Design review of the part built by this model. Coordinates are the model's own, in mm. A direction names the side the tool comes from. Coordinates: 2 decimals unless noted, no trailing zeros. Write each loop counter-clockwise with the first axis right and the second up, starting at its lowest first coordinate (ties: lowest second). Pieces come first, ordered by that corner, then holes. Notation, with made-up numbers: (11, 36) -> (51, 36) arc R10 ccw to (51, 51) -> close; hole circle Ø9 at (30.5, 79.25). An arc over 180 degrees is marked (long way). Answer in a Markdown table with one row per item. Add a question column.
Item 1: Clearance check with flat-ended pins moving along their axes: P1, Ø3.5, axis at x = 11.5, z = 6.5, coming from the -Y side; P2, Ø0.9, axis at x = -3.5, y = -0.5, coming from the -Z side; P3, Ø2, axis at x = -18.5, z = 1.5, coming from the -Y side; P4, Ø4, axis at x = -2.5, z = 1.5, coming from the -Y side. State where each tip first meets the part, or that it passes through.
Item 2: Take a section at A-A, the plane x = -11.5. Write out the cut boundary in (y, z), and give its area (3 significant figures).
Item 3: Take a section at B-B, the plane y = -1. Write out the cut boundary in (x, z).
Item 4: For faces 5 (the face through (-26, 2, 6)), 6 (the face through (-20.62, 0.44, 3.8)), 7 (the face through (-8.324, -2.958, 4.701)), list the 3-axis set-ups (+Z, -Z, +X, -X, +Y, -Y) from which the entire face can be reached by the end or side of a thin tool; tool diameter is ignored.
Item 5: Take a section at C-C, the plane z = 12.25. Write out the cut boundary in (x, y).
Item 6: Draft analysis for pull direction Z (two halves, no side actions). For faces 1 (the face through (-5, 0, 13)), 2 (the face through (-5.88, -4.9, 6.41)), 3 (the face through (11, -1, 10.15)), 4 (the face through (14.646, -1.479, 8.351)), state which applies: released by +Z, released by -Z, zero draft, split by the parting line, or undercut.
Item 7: To check wall thickness, follow line 1 (Z direction, x = -11.5, y = 1.05); line 2 (Z direction, x = 13, y = -1.5); line 3 (X direction, y = -1, z = 6.75). State the ranges of each line that lie inside material, in increasing order.
Item 8: Take a section at D-D, the plane x = 11.5. Write out the cut boundary in (y, z).
from build123d import *

# Parameters (mm, degrees)
F0_R     = 1.45
F1_DEPTH = 13
F2_R     = 2.15
F3_DEPTH = 9.001
F4_DEPTH = 3
F5_DEPTH = 7.7


with BuildPart() as f1:
    # F0 (on Top) → F1 (new body)
    with BuildSketch(Plane.XY):
        with BuildLine():
            Line((17, -3), (17, 3))
            Line((17, 3), (-26, 3))
            Line((-26, 3), (-26, 0))
            ThreePointArc((-26, 0), (-25.2642971497, -2.3117880782), (-23.3278179407, -3.7731816172))
            Line((-23.3278179407, -3.7731816172), (-17, -6))
            Line((-17, -6), (-9, -6))
            Line((-9, -6), (-2.6721820593, -3.7731816172))
            ThreePointArc((-2.6721820593, -3.7731816172), (-1.9759531619, -3.4501064327), (-1.3542486889, -3))
            Line((-1.3542486889, -3), (17, -3))
        make_face()
        with Locations((-22, 0)):
            Circle(F0_R, mode=Mode.SUBTRACT)
        with Locations((-4, 0)):
            Circle(F0_R, mode=Mode.SUBTRACT)
        with Locations((-22, 0)):
            Circle(F0_R)
        with Locations((-4, 0)):
            Circle(F0_R)
    extrude(amount=F1_DEPTH)

    # F2 (on face) → F3 (cut, through all)
    with BuildSketch(Plane(origin=(0, 3, 0), x_dir=(-1, 0, 0), z_dir=(0, 1, 0))):
        Polygon((-9.3926715175, 10.15), (-13.6073284825, 10.15), (-15.7146569651, 6.5), (-13.6073284825, 2.85), (-9.3926715175, 2.85), (-7.2853430349, 6.5), align=None)
        with Locations((-11.5, 6.5)):
            Circle(F2_R, mode=Mode.SUBTRACT)
        Polygon((7.2853430349, 6.5), (9.3926715175, 2.85), (13.6073284825, 2.85), (15.7146569651, 6.5), (13.6073284825, 10.15), (9.3926715175, 10.15), align=None)
        with Locations((11.5, 6.5)):
            Circle(F2_R, mode=Mode.SUBTRACT)
        with Locations((-11.5, 6.5)):
            Circle(F2_R)
        with Locations((11.5, 6.5)):
            Circle(F2_R)
    extrude(amount=-F3_DEPTH, mode=Mode.SUBTRACT)

    # F2 (on face) → F4 (join)
    with BuildSketch(Plane(origin=(0, 3, 0), x_dir=(-1, 0, 0), z_dir=(0, 1, 0))):
        Polygon((-9.3926715175, 10.15), (-13.6073284825, 10.15), (-15.7146569651, 6.5), (-13.6073284825, 2.85), (-9.3926715175, 2.85), (-7.2853430349, 6.5), align=None)
        with Locations((-11.5, 6.5)):
            Circle(F2_R, mode=Mode.SUBTRACT)
        Polygon((7.2853430349, 6.5), (9.3926715175, 2.85), (13.6073284825, 2.85), (15.7146569651, 6.5), (13.6073284825, 10.15), (9.3926715175, 10.15), align=None)
        with Locations((11.5, 6.5)):
            Circle(F2_R, mode=Mode.SUBTRACT)
    extrude(amount=-F4_DEPTH)

    # F0 (on Top) → F5 (cut)
    with BuildSketch(Plane.XY):
        with Locations((-4, 0)):
            Circle(F0_R)
        with Locations((-22, 0)):
            Circle(F0_R)
    extrude(amount=F5_DEPTH, mode=Mode.SUBTRACT)


solid = f1.part
Answers:
| question | item | result |
|---|---|---|
| 1 | P1 | passes through |
| 1 | P2 | stops at z = 7.7 |
| 1 | P3 | stops at y = -5.82 |
| 1 | P4 | stops at y = -4.42 |
| 2 | outline | (-6, 0) -> (3, 0) -> (3, 4.35) -> (0, 4.35) -> (0, 2.85) -> (-6, 2.85) -> close; (-6, 10.15) -> (0, 10.15) -> (0, 8.65) -> (3, 8.65) -> (3, 13) -> (-6, 13) -> close |
| 2 | area | 60.3 mm^2 |
| 3 | outline | (-25.87, 0) -> (-23.05, 0) -> (-23.05, 7.7) -> (-20.95, 7.7) -> (-20.95, 0) -> (-5.05, 0) -> (-5.05, 7.7) -> (-2.95, 7.7) -> (-2.95, 0) -> (17, 0) -> (17, 13) -> (-25.87, 13) -> close; hole (-15.71, 6.5) -> (-13.61, 2.85) -> (-9.39, 2.85) -> (-7.29, 6.5) -> (-9.39, 10.15) -> (-13.61, 10.15) -> close; hole (7.29, 6.5) -> (9.39, 2.85) -> (13.61, 2.85) -> (15.71, 6.5) -> (13.61, 10.15) -> (9.39, 10.15) -> close |
| 4 | face 5 | +Z, -Z, -X, +Y, -Y |
| 4 | face 6 | -Z |
| 4 | face 7 | -Y |
| 5 | outline | (-26, 0) arc R4 ccw to (-23.33, -3.77) -> (-17, -6) -> (-9, -6) -> (-2.67, -3.77) arc R4 ccw to (-1.35, -3) -> (17, -3) -> (17, 3) -> (-26, 3) -> close |
| 6 | face 1 | released by +Z |
| 6 | face 2 | zero draft |
| 6 | face 3 | undercut |
| 6 | face 4 | undercut |
| 7 | line 1 | z = 0 to 4.35, 8.65 to 13 |
| 7 | line 2 | z = 0 to 2.85, 10.15 to 13 |
| 7 | line 3 | x = -25.87 to -23.05, -20.95 to -15.57, -7.43 to -5.05, -2.95 to 7.43, 15.57 to 17 |
| 8 | outline | (-3, 0) -> (3, 0) -> (3, 4.35) -> (0, 4.35) -> (0, 2.85) -> (-3, 2.85) -> close; (-3, 10.15) -> (0, 10.15) -> (0, 8.65) -> (3, 8.65) -> (3, 13) -> (-3, 13) -> close |
